Geometry: final body of the model. Coordinates: model frame, mm. Face numbers are marked on the shaded views. A direction names the side the tool comes from. Give positions to 0.01 mm unless a question says otherwise; leave off trailing zeros. Write each loop counter-clockwise with the first axis right and the second up, starting at its lowest first coordinate (ties: lowest second). Pieces come first, ordered by that corner, then holes. Notation, with made-up numbers: M -14,-1 L 36,-1 A19 cw 36,28 Z; hole C 89,69 d7. An arc over 180 degrees is marked long. Answer as a JSON object with one key per item and string values.
from build123d import *

# Parameters (mm, degrees)
SKETCH1_R           = 23.8275
SKETCH1_R_2         = 16.8275
BOSS_EXTRUDE1_DEPTH = 25
SKETCH2_W           = 25
SKETCH2_H           = 7
BOSS_EXTRUDE2_DEPTH = 70
SKETCH3_W           = 11
SKETCH3_H           = 30
BOSS_EXTRUDE3_DEPTH = 40
SKETCH4_W           = 8.4
SKETCH4_H           = 8.525
CUT_EXTRUDE1_DEPTH  = 1
SKETCH5_W           = 9
SKETCH5_H           = 18.25
CUT_EXTRUDE2_DEPTH  = 1
FILLET1_R           = 0.5
FILLET2_R           = 1
FILLET3_R           = 2
FILLET4_R           = 2
FILLET6_R           = 1


with BuildPart() as part:
    # Sketch1 → Boss-Extrude1 (new body)
    with BuildSketch(Plane(origin=(0, 0, 0), x_dir=(0, 0, -1), z_dir=(1, 0, 0))):
        Circle(SKETCH1_R)
        Circle(SKETCH1_R_2, mode=Mode.SUBTRACT)
    extrude(amount=BOSS_EXTRUDE1_DEPTH)

    # Sketch2 → Boss-Extrude2 (add)
    with BuildSketch(Plane(origin=(0, 0, 0), x_dir=(1, 0, 0), z_dir=(0, 1, 0))):
        with Locations((12.5, -20.3275)):
            Rectangle(SKETCH2_W, SKETCH2_H)
    extrude(amount=BOSS_EXTRUDE2_DEPTH)

    # Sketch3 → Boss-Extrude3 (add)
    with BuildSketch(Plane(origin=(0, 0, 16.8275), x_dir=(-1, 0, 0), z_dir=(0, 0, -1))):
        with Locations((-5.5, 55)):
            Rectangle(SKETCH3_W, SKETCH3_H)
    extrude(amount=BOSS_EXTRUDE3_DEPTH)

    # Sketch4 → Cut-Extrude1 (cut)
    with BuildSketch(Plane(origin=(11, 0, 0), x_dir=(0, 0, -1), z_dir=(1, 0, 0))):
        with Locations((18.9725, 50.7375)):
            Rectangle(SKETCH4_W, SKETCH4_H)
        with Locations((18.9725, 59.2625)):
            Rectangle(SKETCH4_W, SKETCH4_H)
    extrude(amount=-CUT_EXTRUDE1_DEPTH, mode=Mode.SUBTRACT)

    # Sketch5 → Cut-Extrude2 (cut)
    with BuildSketch(Plane(origin=(10, 0, 0), x_dir=(0, 0, -1), z_dir=(1, 0, 0))):
        with Locations((18.6725, 55)):
            Rectangle(SKETCH5_W, SKETCH5_H)
    extrude(amount=-CUT_EXTRUDE2_DEPTH, mode=Mode.SUBTRACT)

    # Fillet1
    fillet1_edges = [part.edges().sort_by_distance(p)[0] for p in [
        (9, 55, -23.1725),
    ]]
    fillet(fillet1_edges, radius=FILLET1_R)

    # Fillet2
    fillet2_edges = [part.edges().sort_by_distance(p)[0] for p in [
        (0, 55, -23.1725),
        (5.5, 70, -23.1725),
        (5.5, 40, -23.1725),
    ]]
    fillet(fillet2_edges, radius=FILLET2_R)

    # Fillet3
    fillet3_edges = [part.edges().sort_by_distance(p)[0] for p in [
        (0, 0, 16.8275),
        (25, 0, 16.8275),
    ]]
    fillet(fillet3_edges, radius=FILLET3_R)

    # Fillet4
    fillet4_edges = [part.edges().sort_by_distance(p)[0] for p in [
        (11, 55, 16.8275),
    ]]
    fillet(fillet4_edges, radius=FILLET4_R)

    # Fillet6
    fillet6_edges = [part.edges().sort_by_distance(p)[0] for p in [
        (11.585786438, 70, 16.241713562),
        (25, 43.43482365, 16.8275),
        (19, 70, 16.8275),
        (11, 66.2625, -23.1725),
        (11, 70, -3.6725),
        (11, 69.707106781, -22.879606781),
    ]]
    fillet(fillet6_edges, radius=FILLET6_R)


solid = part.part
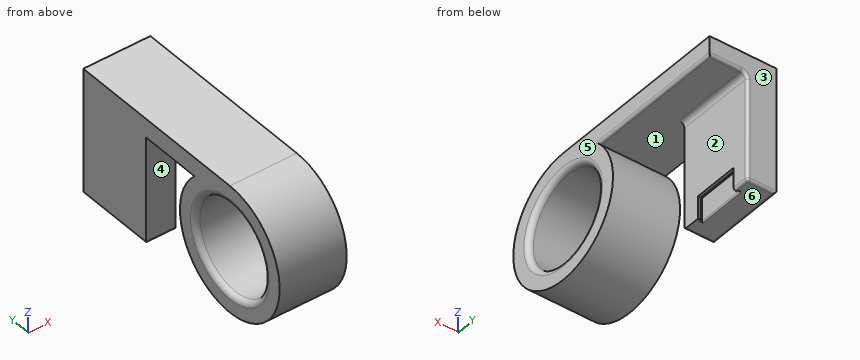
1) Set-up query: the marked faces 4, 5 and 6. Return all of +Z, -Z, +X, -X, +Y, -Y with unobstructed straight access to the full face (end or side cutting, diameter ignored); none if empty.
Geometry check:
{"face 4": "-Z, +X, -X", "face 5": "+Z, -Z, +X, +Y, -Y", "face 6": "-Z, +X, -X, +Y"}
2) Contact query for flat-ended pins moving along their axis: P1, Ø12, axis at x = 4, y = -1.5, coming from the -Z side; P2, Ø14.5, axis at x = 7.5, z = -12, coming from the -Y side; P3, Ø1, axis at x = 15, y = 34, coming from the -Z side; P4, Ø8.5, axis at y = 58.5, z = -9, coming from the +X side. Output: stop coordinate, or through.
Geometry check:
{"P1": "stops at z = -23.83", "P2": "stops at y = -23.35", "P3": "stops at z = 16.83", "P4": "stops at x = 11"}
3) Cut plane B-B on x = 17.75. Return loops of the section in (y, z) (1 decimal), and give its area (3 significant figures).
Geometry check:
{"outline": "M 0,23.8 A23.8 ccw long 16.9,16.8 L 69,16.8 A1 ccw 70,17.8 L 70,23.8 Z; hole C 0,0 d33.7", "area": "1,300 mm2"}
4) Cut plane A-A on z = 0. Return loops of the section in (x, y), and give its area (3 significant figures).
Geometry check:
{"outline": "M 0,-23.83 L 25,-23.83 L 25,-18.83 A2 ccw 23,-16.83 L 2,-16.83 A2 ccw 0,-18.83 Z; M 0,18.83 A2 ccw 2,16.83 L 23,16.83 A2 ccw 25,18.83 L 25,23.83 L 0,23.83 Z; M 0,40 L 11,40 L 11,69 A1 ccw 10,70 L 0,70 Z", "area": "676 mm2"}
5) Cut plane C-C on y = 42. Return loops of the section in (x, z), and give its area (3 significant figures).
Geometry check:
{"outline": "M 0,-22.17 A1 ccw 1,-23.17 L 11,-23.17 L 11,14.83 A2 cw 13,16.83 L 24,16.83 A1 ccw 25,17.83 L 25,23.83 L 0,23.83 Z", "area": "615 mm2"}
6) Pull-direction query (Y, two-part tool) for the marked faces 1, 2 and 3; classes: pulls with the +Y half, pulls with the -Y half, needs draft (parallel to the pull), parting line crosses it, or undercut.
Geometry check:
{"face 1": "undercut", "face 2": "needs draft", "face 3": "pulls with the +Y half"}
7) Line query: line 1 (Z direction, x = 10, y = 0); line 2 (Y direction, x = 9.5, z = 6). Output: solid intervals per line, ascending. Write a range as from..to.
Geometry check:
{"line 1": "z = -23.83..-16.83, 16.83..23.83", "line 2": "y = -23.06..-15.72, 15.72..23.06, 40..70"}
